from build123d import *

# Parameters (mm, degrees)
SKETCH_1_R      = 150
SKETCH_1_R_2    = 2
SKETCH_1_R_3    = 10
EXTRUDE_1_DEPTH = 10


with BuildPart() as part:
    # 草圖1 → 填料-伸長1 (new body)
    with BuildSketch(Plane(origin=(0, 0, 0), x_dir=(1, 0, 0), z_dir=(0, 1, 0))):
        Circle(SKETCH_1_R)
        with Locations((-20, 135)):
            Circle(SKETCH_1_R_2, mode=Mode.SUBTRACT)
        with Locations((20, 135)):
            Circle(SKETCH_1_R_2, mode=Mode.SUBTRACT)
        with Locations((135, 20)):
            Circle(SKETCH_1_R_2, mode=Mode.SUBTRACT)
        with Locations((135, -20)):
            Circle(SKETCH_1_R_2, mode=Mode.SUBTRACT)
        with Locations((20, -135)):
            Circle(SKETCH_1_R_2, mode=Mode.SUBTRACT)
        with Locations((-20, -135)):
            Circle(SKETCH_1_R_2, mode=Mode.SUBTRACT)
        with Locations((-135, -20)):
            Circle(SKETCH_1_R_2, mode=Mode.SUBTRACT)
        with Locations((-135, 20)):
            Circle(SKETCH_1_R_2, mode=Mode.SUBTRACT)
        Circle(SKETCH_1_R_3, mode=Mode.SUBTRACT)
        with Locations((63.889953207, 120.594667707)):
            Circle(SKETCH_1_R_2, mode=Mode.SUBTRACT)
        with Locations((96.110046793, 96.890964003)):
            Circle(SKETCH_1_R_2, mode=Mode.SUBTRACT)
        with Locations((72.493069191, -115.627656377)):
            Circle(SKETCH_1_R_2, mode=Mode.SUBTRACT)
        with Locations((35.855012827, -131.679224083)):
            Circle(SKETCH_1_R_2, mode=Mode.SUBTRACT)
        with Locations((-136.383022398, -4.96701133)):
            Circle(SKETCH_1_R_2, mode=Mode.SUBTRACT)
        with Locations((-131.96505962, 34.78826008)):
            Circle(SKETCH_1_R_2, mode=Mode.SUBTRACT)
    extrude(amount=EXTRUDE_1_DEPTH)


solid = part.part
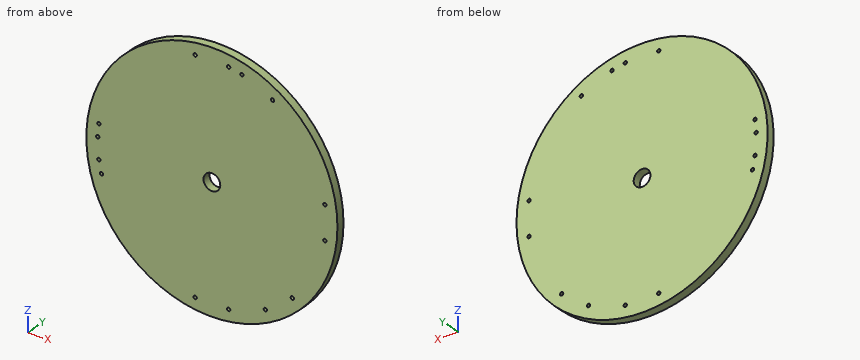
Work out the finished part from the listing and answer in its coordinate system (mm). Coordinates: 2 decimals unless noted, no trailing zeros. Write each loop counter-clockwise with the first axis right and the second up, starting at its lowest first coordinate (ties: lowest second). Pieces come first, ordered by that corner, then holes. Notation, with made-up numbers: (18.5, -9.75) - (61.5, -9.75) arc R16 cw to (61.5, 9.25) - close; hole circle Ø8 at (-9.75, 62.25). An arc over 180 degrees is marked (long way). One line per question, with ' | ' between items.
1) Find section A-A, the plane y = 4. Give the number of separate pieces and of enclosed holes in the cut face, and give its area (3 significant figures).
Checks:
separate pieces: 1 | enclosed holes: 15 | area: 70,200 mm2
2) Consider probe 1 along X at (y, z) = (4.75, 20); probe 2 along Z at (x, y) = (0, 3.25). Determine where each line is inside the solid, lowest interval first. Write a range as [from, to].
Checks:
probe 1: [-148.66, -137], [-133, 133], [137, 148.66] | probe 2: [-150, -10], [10, 150]
3) Flat-ended cylindrical pins translate along their axes: P1, Ø2.5, axis at x = 96.11, z = -96.89, coming from the -Y side; P2, Ø1, axis at x = 92, y = 6, coming from the -Z side; P3, Ø5, axis at y = 1.5, z = 38.5, coming from the -X side; P4, Ø4, axis at x = -47.5, y = 3.5, coming from the -Z side. Find the tip coordinate at first contact, or state that the pin passes through.
Checks:
P1: through | P2: z = -118.86 | P3: x = -145.62 | P4: z = -142.93
4) Find section B-B, the plane z = -126. Determine the outline of the cut face in (x, y), and give its area (3 significant figures).
Checks:
outline: (-81.39, 0) - (81.39, 0) - (81.39, 10) - (-81.39, 10) - close | area: 1,630 mm2
5) Find section C-C, the plane x = 106. Determine the outline of the cut face in (y, z), and give its area (3 significant figures).
Checks:
outline: (0, -106.13) - (10, -106.13) - (10, 106.13) - (0, 106.13) - close | area: 2,120 mm2
